from build123d import *

# Parameters (mm, degrees)
IZIM2_W                     = 50
IZIM2_H                     = 80
Y_KSEKLIK_EKSTR_ZYON1_DEPTH = 12
IZIM7_W                     = 30
IZIM7_H                     = 80
Y_KSEKLIK_EKSTR_ZYON2_DEPTH = 8
Y_KSEKLIK_EKSTR_ZYON3_DEPTH = 58.309518948
IZIM9_R                     = 6.04863379
KES_EKSTR_ZYON2_DEPTH       = 69
RADYUS1_R                   = 2
IZIM10_R                    = 5.458003929
IZIM10_R_2                  = 5.171696766
KES_EKSTR_ZYON3_DEPTH       = 69


with BuildPart() as part:
    # Çizim2 → Yükseklik-Ekstrüzyon1 (new body)
    with BuildSketch(Plane(origin=(0, 0, 0), x_dir=(1, 0, 0), z_dir=(0, 1, 0))):
        with Locations((21.624459622, 0.233673548)):
            Rectangle(IZIM2_W, IZIM2_H)
    extrude(amount=Y_KSEKLIK_EKSTR_ZYON1_DEPTH)

    # Çizim7 → Yükseklik-Ekstrüzyon2 (add)
    with BuildSketch(Plane.XZ):
        with Locations((21.691574622, -0.233673548)):
            Rectangle(IZIM7_W, IZIM7_H)
    extrude(amount=Y_KSEKLIK_EKSTR_ZYON2_DEPTH)

    # Çizim8 → Yükseklik-Ekstrüzyon3 (add, along a direction that is not the sketch's normal)
    with BuildSketch(Plane(origin=(46.624459622, 0, 0), x_dir=(0, 0, -1), z_dir=(1, 0, 0))):
        with BuildLine():
            Line((21.233673548, 12), (30.233673548, 12))
            ThreePointArc((30.233673548, 12), (15.233673548, 27), (0.233673548, 12))
            Line((0.233673548, 12), (9.233673548, 12))
            ThreePointArc((9.233673548, 12), (15.233673548, 18), (21.233673548, 12))
        make_face()
    extrude(amount=-Y_KSEKLIK_EKSTR_ZYON3_DEPTH, dir=(0.8574929257125442, 0, -0.5144957554275265))

    # Çizim9 → Kes-Ekstrüzyon2 (cut, along a direction that is not the sketch's normal)
    with BuildSketch(Plane(origin=(46.624459622, 0, 0), x_dir=(0, 0, -1), z_dir=(1, 0, 0))):
        with Locations((15.282307338, 12)):
            Circle(IZIM9_R)
    extrude(amount=-KES_EKSTR_ZYON2_DEPTH, dir=(0.8574929257125442, 0, -0.5144957554275265), mode=Mode.SUBTRACT)

    # Radyus1
    radyus1_edges = [part.edges().sort_by_distance(p)[0] for p in [
        (21.624459622, 12, 14.766326452),
        (21.624459622, 12, -15.233673548),
    ]]
    fillet(radyus1_edges, radius=RADYUS1_R)

    # Çizim10 → Kes-Ekstrüzyon3 (cut)
    with BuildSketch(Plane(origin=(0, 12, 0), x_dir=(1, 0, 0), z_dir=(0, 1, 0))):
        with Locations(Location((21.624459622, -29.766326452, 0), (0, 0, 270))):
            Circle(IZIM10_R)
        with Locations(Location((21.624459622, 30.233673548, 0), (0, 0, 270))):
            Circle(IZIM10_R_2)
    extrude(amount=-KES_EKSTR_ZYON3_DEPTH, mode=Mode.SUBTRACT)


solid = part.part
The model under review builds one solid part; all positions refer to its coordinate system, in mm. A direction names the side the tool comes from. Round coordinates to 2 decimals unless told otherwise and drop trailing zeros. Write each loop counter-clockwise with the first axis right and the second up, starting at its lowest first coordinate (ties: lowest second). Pieces come first, ordered by that corner, then holes. Notation, with made-up numbers: M 86.5,2 L 120.5,2 A19 cw 120.5,27 Z; hole C -31,-11 d2. An arc over 180 degrees is marked long. Use a Markdown table: item, result. Add a question column.
Q1. To check wall thickness, follow line 1 (Z direction, x = 19, y = 3); line 2 (Z direction, x = 17, y = 10); line 3 (Z direction, x = 25, y = 3). State the ranges of each line that lie inside material, in increasing order.
Q2. We need section B-B, the plane y = -2. State the section outline as (x, z) points, plus the area to 3 significant figures.
Q3. We need section A-A, the plane y = 4. State the section outline as (x, z) points, plus the area to 3 significant figures.
Q4. The part is to be moulded in two halves that separate along Z. For faces 1 (the face through (21, 4, 39.766)), 2 (the face through (42, 0, -1)), 3 (the face through (19.64, 2.14, -25.46)), 4 (the face through (21.864, 2.14, 24.314)), say which applies: pulls with the +Z half, pulls with the -Z half, needs draft (parallel to the pull), parting line crosses it, or undercut.
Q5. Machinability: for faces 5 (the face through (27, 12, 25)), 6 (the face through (36.692, -4, -1)), 7 (the face through (6.692, -4, -1)), 8 (the face through (16, 12, -26)), which of the approach directions +Z, -Z, +X, -X, +Y, -Y give a long, thin tool a straight path to every point of the face, cutting with its end or side? Answer none if there is none.
Q6. Insertion check: pin 1 (4 mm diameter, centred on y = -3.5, z = -17, fed in from -X); pin 2 (10 mm diameter, centred on x = 28, y = 22, fed in from -Z); pin 3 (4 mm diameter, centred on y = -5.5, z = 8, fed in from +X); pin 4 (2 mm diameter, centred on y = 13.5, z = 31, fed in from -X). Each pin has a flat end and moves straight along its axis. Give the tip position at first contact, or say it passes through.
Findings below:
| question | item | result |
|---|---|---|
| 1 | line 1 | z = -40.23 to -34.69, -25.78 to 24.98, 34.55 to 39.77 |
| 1 | line 2 | z = -40.23 to -32.55, -27.92 to -3.22, 8.2 to 26.87, 32.67 to 39.77 |
| 1 | line 3 | z = -40.23 to -34.15, -26.32 to 25.48, 34.06 to 39.77 |
| 2 | outline | M 6.69,-40.23 L 36.69,-40.23 L 36.69,39.77 L 6.69,39.77 Z; hole C 21.62,29.77 d10.92; hole C 21.62,-30.23 d10.34 |
| 2 | area | 2,220 mm² |
| 3 | outline | M -3.38,-40.23 L 46.62,-40.23 L 46.62,39.77 L -3.38,39.77 Z; hole C 21.62,29.77 d10.92; hole C 21.62,-30.23 d10.34 |
| 3 | area | 3,820 mm² |
| 4 | face 1 | pulls with the +Z half |
| 4 | face 2 | needs draft |
| 4 | face 3 | undercut |
| 4 | face 4 | undercut |
| 5 | face 5 | +Z, +X, +Y |
| 5 | face 6 | +Z, -Z, +X, -Y |
| 5 | face 7 | +Z, -Z, -X, -Y |
| 5 | face 8 | -Z, -X, +Y |
| 6 | pin 1 | stops at x = 6.69 |
| 6 | pin 2 | stops at z = -19.73 |
| 6 | pin 3 | stops at x = 36.69 |
| 6 | pin 4 | passes through |
